Design review of the part built by this model. Coordinates are the model's own, in mm. A direction names the side the tool comes from. Round coordinates to 2 decimals unless told otherwise and drop trailing zeros. Order: outer loops, then holes, each group sorted by start corner. A loop starts at its lowest first (then second) coordinate and runs counter-clockwise, first axis right, second up. Notation, with made-up numbers: (67, -4) - (109, -4) arc R13 cw to (109, 16) - close; hole circle Ø10 at (-20.5, 47). An arc over 180 degrees is marked (long way). Use CSV: the item, a comma, the result in double quotes.
from build123d import *

# Parameters (mm, degrees)
PIED_GAUCHE_SYM_TRIQUE_START = 8.25
PIED_GAUCHE_SYM_TRIQUE_DEPTH = 13.5
ESQUISSE2_W                  = 127.532024566
ESQUISSE2_H                  = 119.503632389
ENL_V_MAT_EXTRU_3_DEPTH      = 302.826111243
ESQUISSE3_W                  = 31.738465923
ESQUISSE3_H                  = 10.347254195
ENL_V_MAT_EXTRU_5_DEPTH      = 207.107541608


# Read off the part's stored shape, not the designer's step: pied_gauche_Symétrique
with BuildPart() as part:
    # pied_gauche_Symétrique outline → pied_gauche_Symétrique (new body)
    with BuildSketch(Plane(origin=(0, 0, 0), x_dir=(1, 0, 0), z_dir=(0, 1, 0)).offset(PIED_GAUCHE_SYM_TRIQUE_START)):
        with BuildLine():
            add(Edge.make_bspline(
                [(37.478644966, -252.078923217), (36.315942048, -246.147042601), (34.178554605, -240.439587675)],
                knots=[0.172395677, 0.172395677, 0.172395677, 1, 1, 1], degree=2))
            ThreePointArc((37.478644966, -252.078923217), (68.296716845, -277.385748803), (95.718365725, -248.433337016))
            ThreePointArc((95.718365725, -248.433337016), (95.727304168, -248.184441724), (95.749998935, -247.936422149))
            Line((95.749998935, -247.936422149), (116.839136919, -71.443633134))
            ThreePointArc((116.839136919, -71.443633134), (100.314842401, -61.417925092), (84.153017918, -72.018045866))
            ThreePointArc((84.153017918, -72.018045866), (74.728050938, -68.392019497), (65.697628344, -72.911924095))
            ThreePointArc((65.697628344, -72.911924095), (48.169524668, -72.986859822), (37.57616681, -86.951844718))
            add(Edge.make_bspline(
                [(37.57616681, -86.951844718), (36.224938138, -91.89952807), (34.78531821, -96.822767534)],
                knots=[0.221662646, 0.221662646, 0.221662646, 1, 1, 1], degree=2))
            ThreePointArc((34.78531821, -96.822767534), (21.501008197, -168.576334761), (34.178554605, -240.439587675))
        make_face()
    extrude(amount=PIED_GAUCHE_SYM_TRIQUE_DEPTH)

    # Esquisse2 → Enlèv. mat.-Extru.3 (cut, through all)
    with BuildSketch(Plane(origin=(0, 0, 0), x_dir=(1, 0, 0), z_dir=(0, 1, 0))):
        with Locations((63.766012283, -228.143835691)):
            Rectangle(ESQUISSE2_W, ESQUISSE2_H)
    extrude(amount=ENL_V_MAT_EXTRU_3_DEPTH, mode=Mode.SUBTRACT)

    # Esquisse3 → Enlèv. mat.-Extru.5 (cut, through all)
    with BuildSketch(Plane(origin=(0, 0, 0), x_dir=(0, 0, -1), z_dir=(1, 0, 0))):
        with Locations((-154.261252458, 9.826372903)):
            Rectangle(ESQUISSE3_W, ESQUISSE3_H)
    extrude(amount=ENL_V_MAT_EXTRU_5_DEPTH, mode=Mode.SUBTRACT)


solid = part.part
1) We need section B-B (z = 114). Give the boundary of the cut face in (x, y).
Data:
outline,"(29.13, 8.25) - (111.75, 8.25) - (111.75, 21.75) - (29.13, 21.75) - close"
2) For faces 4 (the face through (63, 18, 168.392)), 5 (the face through (66, 12, 138.392)), list the 3-axis set-ups (+Z, -Z, +X, -X, +Y, -Y) from which the entire face can be reached by the end or side of a thin tool; tool diameter is ignored.
Data:
face 4,"+Z, +X, -X, +Y, -Y"
face 5,"+Z, +X, -X, -Y"
3) The part is to be moulded in two halves that separate along X. For faces 1 (the face through (48.398, 14.906, 72.875)), 2 (the face through (26.7, 16.41, 123.55)), 3 (the face through (71, 8.25, 99)), say which applies: +X half, -X half, draft (parallel to the pull), parting line (faces both ways), or undercut.
Data:
face 1,"undercut"
face 2,"-X half"
face 3,"draft"
4) We need section D-D (z = 159.5). Give the boundary of the cut face in (x, y).
Data:
outline,"(21.74, 15) - (106.32, 15) - (106.32, 21.75) - (21.74, 21.75) - close"
5) To check wall thickness, follow L1, parallel to Z at x = 56, y = 11; L2, parallel to Y at x = 30, z = 164; L3, parallel to Z at x = 100.5, y = 14.5. State the ranges of each line that lie inside material, in increasing order. Write a range as from..to.
Data:
L1,"z = 70.93..138.39"
L2,"y = 15..21.75"
L3,"z = 61.42..138.39"
6) We need section A-A (x = 33.5). Give the boundary of the cut face in (y, z).
Data:
outline,"(8.25, 100.31) - (21.75, 100.31) - (21.75, 168.39) - (15, 168.39) - (15, 138.39) - (8.25, 138.39) - close"
7) Insertion check: pin 1 Ø3 at (y, z) = (15, 107.5) entering from -X; pin 2 Ø1.5 at (y, z) = (19, 131.5) entering from +X; pin 3 Ø24 at (x, z) = (55.5, 149.5) entering from -Y; pin 4 Ø4 at (y, z) = (17.5, 137.5) entering from +X. Each pin has a flat end and moves straight along its axis. Give the tip position at first contact, or say it passes through.
Data:
pin 1,"stops at x = 30.61"
pin 2,"stops at x = 109.75"
pin 3,"stops at y = 8.25"
pin 4,"stops at x = 109.19"
8) We need section C-C (x = 104). Give the boundary of the cut face in (y, z), then the cut area to 3 significant figures.
Data:
outline,"(8.25, 61.73) - (21.75, 61.73) - (21.75, 168.39) - (15, 168.39) - (15, 138.39) - (8.25, 138.39) - close"
area,"1,240 mm2"
